Answer from the drawing. Dimensions are ordinates in mm from the lowest x, y and z of the part. Give positions to 0.01 mm unless a question says otherwise; leave off trailing zeros. Loops run counter-clockwise (first coordinate to the right, second up) from the corner with the lowest first, then second, coordinate; pieces in that order, holes last. Notation, with made-up numbers: (15.5, -14) - (32.5, -14) arc R25 cw to (32.5, 5) - close; hole circle Ø1 at (26.5, 42.25). An arc over 180 degrees is marked (long way). Answer as CSV lines item,"result". Start each with the question number.
1) A cutting plane is placed at A-A (z = 47.5). Determine the outline of the cut face in (x, y), and give its area (3 significant figures).
2) A cutting plane is placed at C-C (x = 1.25). Determine the outline of the cut face in (y, z).
3) A cutting plane is placed at B-B (y = 35.5). Determine the outline of the cut face in (x, z), and give its area (3 significant figures).
4) Find the intervals of material crossed by line 1 along Y through (x, z) = (1.1, 47.5); line 2 along Y through (x, z) = (2.4, 45); line 3 along Z through (x, y) = (1.55, 81), in increasing order.
5) A cutting plane is placed at D-D (y = 116). Determine the outline of the cut face in (x, z).
6) Flat-ended cylindrical pins translate along their axes: pin 1 (1.5 mm diameter, centred on x = 1, y = 168, fed in from -Z); pin 2 (1.5 mm diameter, centred on x = 2, y = 74.5, fed in from +Z); pin 3 (1.5 mm diameter, centred on x = 2.5, z = 53, fed in from +Y); pin 4 (1.5 mm diameter, centred on x = 1, z = 58, fed in from -Y). Find the tip coordinate at first contact, or state that the pin passes through.
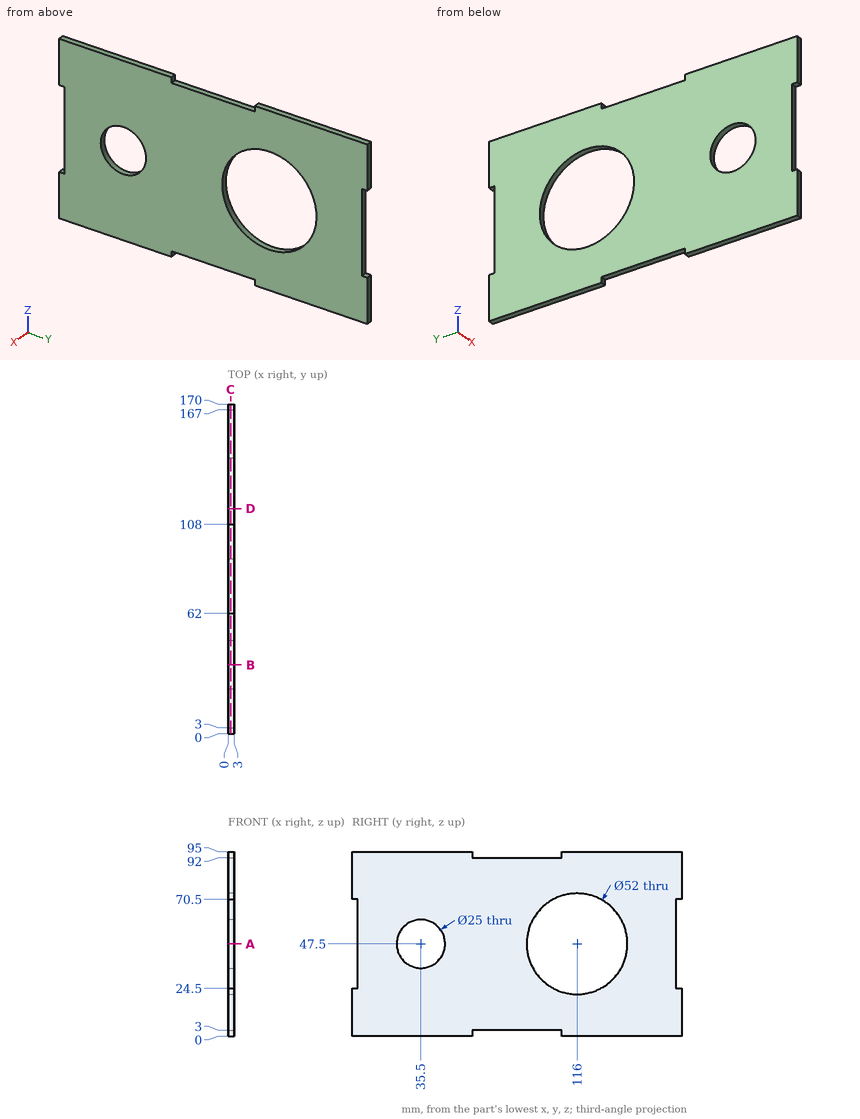
Ans:
1,outline,"(0, 3) - (3, 3) - (3, 23) - (0, 23) - close; (0, 48) - (3, 48) - (3, 90) - (0, 90) - close; (0, 142) - (3, 142) - (3, 167) - (0, 167) - close"
1,area,"261 mm2"
2,outline,"(0, 0) - (62, 0) - (62, 3) - (108, 3) - (108, 0) - (170, 0) - (170, 24.5) - (167, 24.5) - (167, 70.5) - (170, 70.5) - (170, 95) - (108, 95) - (108, 92) - (62, 92) - (62, 95) - (0, 95) - (0, 70.5) - (3, 70.5) - (3, 24.5) - (0, 24.5) - close; hole circle Ø25 at (35.5, 47.5); hole circle Ø52 at (116, 47.5)"
3,outline,"(0, 0) - (3, 0) - (3, 35) - (0, 35) - close; (0, 60) - (3, 60) - (3, 95) - (0, 95) - close"
3,area,"210 mm2"
4,line 1,"3 to 23, 48 to 90, 142 to 167"
4,line 2,"3 to 23.25, 47.75 to 90.12, 141.88 to 167"
4,line 3,"3 to 92"
5,outline,"(0, 0) - (3, 0) - (3, 21.5) - (0, 21.5) - close; (0, 73.5) - (3, 73.5) - (3, 95) - (0, 95) - close"
6,pin 1,"z = 0"
6,pin 2,"z = 92"
6,pin 3,"y = 167"
6,pin 4,"y = 3"
